Could you check a few things on this model? Use its own coordinates, in mm. A direction names the side the tool comes from. Coordinates: 2 decimals unless noted, no trailing zeros. Write each loop counter-clockwise with the first axis right and the second up, starting at its lowest first coordinate (ties: lowest second). Pieces come first, ordered by that corner, then holes.
```python
from build123d import *

# Parameters (mm, degrees)
BOSS_EXTRUDE1_DEPTH = 1.5
SKETCH2_W           = 3
SKETCH2_H           = 15
BOSS_EXTRUDE2_DEPTH = 1.5
FILLET1_R           = 4


with BuildPart() as part:
    # Sketch1 → Boss-Extrude1 (new, symmetric)
    with BuildSketch(Plane(origin=(0, 0, 0), x_dir=(1, 0, 0), z_dir=(0, 1, 0))):
        Polygon((-10, 17.5), (10, -17.5), (-10, -17.5), align=None)
    extrude(amount=BOSS_EXTRUDE1_DEPTH, both=True)

    # Sketch2 → Boss-Extrude2 (add, symmetric)
    with BuildSketch(Plane(origin=(0, 0, 0), x_dir=(1, 0, 0), z_dir=(0, 1, 0))):
        with Locations((-11.5, -7)):
            Rectangle(SKETCH2_W, SKETCH2_H)
    extrude(amount=BOSS_EXTRUDE2_DEPTH, both=True)

    # Fillet1
    fillet1_edges = [part.edges().sort_by_distance(p)[0] for p in [
        (-10, 0, -17.5),
    ]]
    fillet(fillet1_edges, radius=FILLET1_R)


solid = part.part
```
Item 1: I want a section at B-B, the plane x = -2. List the corners of the cut face in (y, z) for me, then the cut area to 3 significant figures.
Item 2: I want a section at A-A, the plane y = 0.65. List the corners of the cut face in (x, z) for me, then the cut area to 3 significant figures.
Item 3: I want a section at C-C, the plane z = 7.25. List the corners of the cut face in (x, y) for me.
Item 4: If I drill on line 1 along Z through (x, y) = (-12, 1); line 2 along Z through (x, y) = (-9.5, 0.1); line 3 along X through (y, z) = (0.4, -4.5), over which ranges is the centre line in solid material (lowest first)?
Item 5: Which directions (+Z, -Z, +X, -X, +Y, -Y) give clear straight access to the entire face, cutting with the end or side of a thin tool? Please do faces 1 (the flat face through (-13, 0, 7)), 2 (the flat face through (-12, 0, -0.5)), 3 (the flat face through (-10, 0, 16)).
Item 6: Will these pins go through, and if not, where does the flat tip stop? pin 1 Ø0.9 at (x, y) = (-11, 0) entering from -Z; pin 2 Ø1.5 at (x, y) = (-11.5, -0.5) entering from +Z; pin 3 Ø2 at (x, z) = (5, 4) entering from +Y.
Taken from the geometry:
1. outline: (-1.5, -3.5) - (1.5, -3.5) - (1.5, 17.5) - (-1.5, 17.5) - close
1. area: 63.0 mm2
2. outline: (-13, -0.5) - (-10, -0.5) - (-10, -2.44) arc R4 ccw to (-2.53, -4.42) - (10, 17.5) - (-10, 17.5) - (-10, 14.5) - (-13, 14.5) - close
2. area: 356 mm2
3. outline: (-13, -1.5) - (4.14, -1.5) - (4.14, 1.5) - (-13, 1.5) - close
4. line 1: z = -0.5 to 14.5
4. line 2: z = -4.37 to 17.5
4. line 3: x = -9.43 to -2.57
5. face 1: +Z, -Z, -X, +Y, -Y
5. face 2: -Z, -X, +Y, -Y
5. face 3: +Z, -X, +Y, -Y
6. pin 1: stops at z = -0.5
6. pin 2: stops at z = 14.5
6. pin 3: passes through
